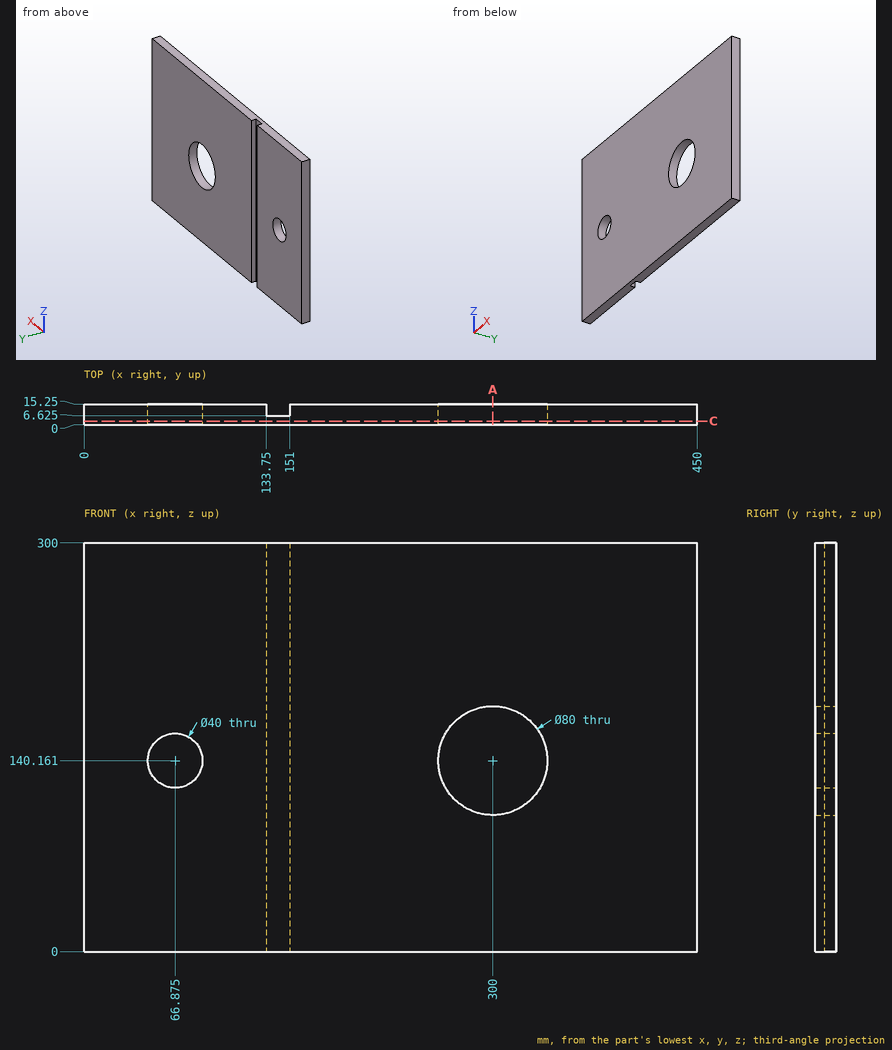
Print and shaded views of the part. All mm, measured from the part's lowest x, y and z. Coordinates: 2 decimals unless noted, no trailing zeros. Order: outer loops, then holes, each group sorted by start corner. A loop starts at its lowest first (then second) coordinate and runs counter-clockwise, first axis right, second up. Notation, with made-up numbers: (33, 46.5) -> (42, 46.5) arc R11 cw to (42, 64.5) -> close; hole circle Ø5 at (49.5, 86). An arc over 180 degrees is marked (long way). Answer as a JSON object with one key per item and string values. Group by question number.
1) Cut at C-C, the plane y = 2.75. Write the cut outline in (x, z) (1 decimal), then the cut area to 3 significant figures.
2) Flat gauge pin, fed straight in: pin 1 (5 mm diameter, centred on x = 140.5, z = 182.5, fed in from +Y) (3 decimals). Where does the tip first touch, or does it go through?
3) Drill centre lines: L1, parallel to X at y = 7.75, z = 145; L2, parallel to X at y = 5.75, z = 123 (1 decimal); L3, parallel to Z at x = 300, y = 10. Where is each one in solid material? Low to high.
4) Cut at A-A, the plane x = 300. Write the cut outline in (y, z), then the cut area to 4 significant figures.
Check values:
{
 "1": {"outline": "(0, 0) -> (450, 0) -> (450, 300) -> (0, 300) -> close; hole circle Ø40 at (66.9, 140.2); hole circle Ø80 at (300, 140.2)", "area": "129,000 mm²"},
 "2": {"pin 1": "stops at y = 6.625"},
 "3": {"L1": "x = 0 to 47.47, 86.28 to 133.75, 151 to 260.29, 339.71 to 450", "L2": "x = 0 to 56.6, 77.1 to 263.9, 336.1 to 450", "L3": "z = 0 to 100.16, 180.16 to 300"},
 "4": {"outline": "(0, 0) -> (15.25, 0) -> (15.25, 100.16) -> (0, 100.16) -> close; (0, 180.16) -> (15.25, 180.16) -> (15.25, 300) -> (0, 300) -> close", "area": "3,355 mm²"}
}
